from build123d import *

# Parameters (mm, degrees)
SKETCH1_W           = 75
SKETCH1_H           = 84
BOSS_EXTRUDE1_DEPTH = 12.5
SKETCH2_W           = 6.25
SKETCH2_H           = 22
CUT_EXTRUDE1_DEPTH  = 12
SKETCH3_R           = 2.25
CUT_EXTRUDE2_DEPTH  = 87.863398506
SKETCH4_W           = 75
SKETCH4_H           = 20
CUT_EXTRUDE3_DEPTH  = 3.5


with BuildPart() as part:
    # Sketch1 → Boss-Extrude1 (new body)
    with BuildSketch(Plane(origin=(0, 0, 0), x_dir=(1, 0, 0), z_dir=(0, 1, 0))):
        Rectangle(SKETCH1_W, SKETCH1_H)
    extrude(amount=BOSS_EXTRUDE1_DEPTH)

    # Sketch2 → Cut-Extrude1 (cut)
    with BuildSketch(Plane.XZ):
        with Locations((24.375, 0)):
            Rectangle(SKETCH2_W, SKETCH2_H)
    extrude(amount=-CUT_EXTRUDE1_DEPTH, mode=Mode.SUBTRACT)

    # Sketch3 → Cut-Extrude2 (cut, through all)
    with BuildSketch(Plane(origin=(37.5, 0, 0), x_dir=(0, 0, -1), z_dir=(1, 0, 0))):
        with Locations((-6, 6)):
            Circle(SKETCH3_R)
        with Locations((6, 6)):
            Circle(SKETCH3_R)
    extrude(amount=-CUT_EXTRUDE2_DEPTH, mode=Mode.SUBTRACT)

    # Sketch4 → Cut-Extrude3 (cut)
    with BuildSketch(Plane(origin=(0, 12.5, 0), x_dir=(1, 0, 0), z_dir=(0, 1, 0))):
        with Locations((0, 32)):
            Rectangle(SKETCH4_W, SKETCH4_H)
        with Locations((0, -32)):
            Rectangle(SKETCH4_W, SKETCH4_H)
    extrude(amount=-CUT_EXTRUDE3_DEPTH, mode=Mode.SUBTRACT)


solid = part.part
For this review, take the finished solid that the model builds, in its own axes (mm). A direction names the side the tool comes from. Round coordinates to 2 decimals unless told otherwise and drop trailing zeros. Order: outer loops, then holes, each group sorted by start corner. A loop starts at its lowest first (then second) coordinate and runs counter-clockwise, first axis right, second up. Notation, with made-up numbers: (-39.5, 54) -> (19.5, 54) arc R31 ccw to (19.5, 84) -> close; hole circle Ø3 at (20, -17). An arc over 180 degrees is marked (long way). Write item = value, one per line. Start each with the question number.
1) Take a section at B-B on z = -6. State the section outline as (x, y) points, plus the area to 3 significant figures.
2) Take a section at D-D on y = 10.5. State the section outline as (x, z) points, plus the area to 3 significant figures.
3) Take a section at C-C on x = 4.5. State the section outline as (y, z) points, plus the area to 3 significant figures.
4) To check wall thickness, follow line 1 (Y direction, x = -21.5, z = 6); line 2 (Z direction, x = -12, y = 6.25); line 3 (X direction, y = 9, z = -8). State the ranges of each line that lie inside material, in increasing order. Write a range as from..to.
5) Take a section at A-A on y = 6. State the section outline as (x, z) points, plus the area to 3 significant figures.
6) Insertion check: pin 1 (10 mm diameter, centred on x = 15, z = -32, fed in from +Y); pin 2 (1.8 mm diameter, centred on x = 15, y = 10.5, fed in from -Z); pin 3 (4 mm diameter, centred on y = 6, z = -6, fed in from -X); pin 4 (1 mm diameter, centred on x = -17.5, y = 11, fed in from +Z). Each pin has a flat end and moves straight along its axis. Give the tip position at first contact, or say it passes through.
7) The part is to be moulded in two halves that separate along X. For faces 1 (the face through (37.5, 6, 1)), 2 (the face through (24, 6, 11)), 3 (the face through (-1, 11, 22)), say which applies: +X half, -X half, draft (parallel to the pull), parting line (faces both ways), or undercut.
8) Tool access review of faces 4 (the face through (24, 12, 0)), 5 (the face through (-1, 11, -22)), 6 (the face through (32.57, 6.676, -8.146)), 7 (the face through (-1, 9, 32)): name each direction out of +Z, -Z, +X, -X, +Y, -Y from which nothing blocks a thin tool from reaching the whole face with its end or side.
Verdict:
q1.outline = (-37.5, 0) -> (21.25, 0) -> (21.25, 3.75) -> (-37.5, 3.75) -> close; (-37.5, 8.25) -> (21.25, 8.25) -> (21.25, 12) -> (27.5, 12) -> (27.5, 8.25) -> (37.5, 8.25) -> (37.5, 12.5) -> (-37.5, 12.5) -> close; (27.5, 0) -> (37.5, 0) -> (37.5, 3.75) -> (27.5, 3.75) -> close
q1.area = 553 mm2
q2.outline = (-37.5, -22) -> (37.5, -22) -> (37.5, 22) -> (-37.5, 22) -> close; hole (21.25, -11) -> (27.5, -11) -> (27.5, 11) -> (21.25, 11) -> close
q2.area = 3,160 mm2
q3.outline = (0, -42) -> (9, -42) -> (9, -22) -> (12.5, -22) -> (12.5, 22) -> (9, 22) -> (9, 42) -> (0, 42) -> close; hole circle Ø4.5 at (6, -6); hole circle Ø4.5 at (6, 6)
q3.area = 878 mm2
q4.line_1 = 0..3.75, 8.25..12.5
q4.line_2 = -42..-8.24, -3.76..3.76, 8.24..42
q4.line_3 = -37.5..21.25, 27.5..37.5
q5.outline = (-37.5, -42) -> (37.5, -42) -> (37.5, -8.25) -> (27.5, -8.25) -> (27.5, -11) -> (21.25, -11) -> (21.25, -8.25) -> (-37.5, -8.25) -> close; (-37.5, -3.75) -> (21.25, -3.75) -> (21.25, 3.75) -> (-37.5, 3.75) -> close; (-37.5, 8.25) -> (21.25, 8.25) -> (21.25, 11) -> (27.5, 11) -> (27.5, 8.25) -> (37.5, 8.25) -> (37.5, 42) -> (-37.5, 42) -> close; (27.5, -3.75) -> (37.5, -3.75) -> (37.5, 3.75) -> (27.5, 3.75) -> close
q5.area = 5,540 mm2
q6.pin_1 = 9
q6.pin_2 = -22
q6.pin_3 = through
q6.pin_4 = 22
q7.face_1 = +X half
q7.face_2 = undercut
q7.face_3 = draft
q8.face_4 = -Y
q8.face_5 = -Z, +X, -X, +Y
q8.face_6 = +X, -X
q8.face_7 = +Z, +X, -X, +Y
